For this review, take the finished solid that the model builds, in its own axes (mm). A direction names the side the tool comes from. Give positions to 0.01 mm unless a question says otherwise; leave off trailing zeros. Order: outer loops, then holes, each group sorted by start corner. A loop starts at its lowest first (then second) coordinate and runs counter-clockwise, first axis right, second up. Notation, with made-up numbers: (25, 43.5) - (45, 43.5) arc R15 ccw to (45, 62.5) - close; hole circle Ø10 at (43, 62.25). An arc over 180 degrees is marked (long way). One line per item, written item: value.
```python
from build123d import *

# Parameters (mm, degrees)
F2_R     = 0.2
F4_DEPTH = 5


with BuildPart() as f1:
    # F0 (on Front) → F1 (revolve)
    with BuildSketch(Plane.XZ):
        with BuildLine():
            Line((0, 9.25), (0, 0))
            Line((0, 0), (4, 0))
            Line((4, 0), (4, 10))
            Line((4, 10), (3.75, 10))
            ThreePointArc((3.75, 10), (1.9121323176, 9.439338412), (0, 9.25))
        make_face()
        with BuildLine():
            Line((0, 10), (0, 9.25))
            ThreePointArc((0, 9.25), (1.9121323176, 9.439338412), (3.75, 10))
            Line((3.75, 10), (0, 10))
        make_face()
        with BuildLine():
            Line((3.75, 10), (4, 10))
            ThreePointArc((4, 10), (2.0615528128, 10.7462112512), (0, 11))
            Line((0, 11), (0, 10))
            Line((0, 10), (3.75, 10))
        make_face()
    revolve(axis=Axis((0, 0, 5), (0, 0, -1)))

    # F2
    f2_edges = [f1.edges().sort_by_distance(p)[0] for p in [
        (-4, 0, 10),
    ]]
    fillet(f2_edges, radius=F2_R)

    # F3 (on Top) → F4 (join)
    with BuildSketch(Plane.XY):
        Polygon((-1, 7), (-1, 0), (0, 0), (0, 1), (1, 1), (1, 7), align=None)
        Polygon((1, 0), (0, 0), (0, -1), (7, -1), (7, 1), (1, 1), align=None)
    extrude(amount=F4_DEPTH)


solid = f1.part
```
(1) For P1, Ø3, axis at x = -0.5, y = 4, coming from the -Z side; P2, Ø0.6, axis at x = 0.5, y = 5.5, coming from the +Z side; P3, Ø1.6, axis at y = 5.5, z = 2, coming from the -X side; P4, Ø0.9, axis at y = 5, z = 3.5, coming from the +X side, all flat-tipped, find the tip position at first contact; note any pin that passes through.
Answers below:
P1: stops at z = 0
P2: stops at z = 5
P3: stops at x = -1
P4: stops at x = 1
(2) Take a section at B-B (x = 5). Write out the cut boundary in (y, z), then the cut area to 3 significant figures.
Answers below:
outline: (-1, 0) - (1, 0) - (1, 5) - (-1, 5) - close
area: 10.0 mm^2
(3) Machinability: for faces 1 (the face through (5, -1, 2)), 2 (the face through (1, 5, 2)), 3 (the face through (-1, 5, 2)), which of the approach directions +Z, -Z, +X, -X, +Y, -Y give a long, thin tool a straight path to every point of the face, cutting with its end or side? Answer none if there is none.
Answers below:
face 1: +Z, -Z, +X, -Y
face 2: +Z, -Z, +X, +Y
face 3: +Z, -Z, -X, +Y
(4) Take a section at D-D (z = 5.75). Write out the cut boundary in (x, y), then the cut area to 3 significant figures.
Answers below:
outline: circle Ø8 at (0, 0)
area: 50.3 mm^2
(5) Wall thickness on line 1 (Y direction, x = 4, z = 3.25); line 2 (Z direction, x = 5.5, y = -0.75); line 3 (Y direction, x = -0.75, z = 7.5): over which ranges is each line inside the solid? List them lowest first. Write a range as from..to.
Answers below:
line 1: y = -1..1
line 2: z = 0..5
line 3: y = -3.93..3.93
(6) Take a section at A-A (z = 2.5). Write out the cut boundary in (x, y), then the cut area to 3 significant figures.
Answers below:
outline: (-1, 3.87) arc R4 ccw (long way) to (3.87, -1) - (7, -1) - (7, 1) - (3.87, 1) arc R4 ccw to (1, 3.87) - (1, 7) - (-1, 7) - close
area: 62.4 mm^2
